from build123d import *

# Parameters (mm, degrees)
BOSS_EXTRUDE1_DEPTH = 10
BOSS_EXTRUDE2_DEPTH = 20
BOSS_EXTRUDE3_REACH = 38.449
FILLET1_R           = 1
CUT_EXTRUDE1_DEPTH  = 7


with BuildPart() as part:
    # Sketch1 → Boss-Extrude1 (new body)
    with BuildSketch(Plane(origin=(0, 0, 0), x_dir=(1, 0, 0), z_dir=(0, 1, 0))):
        Polygon((15, 0), (12.135254916, 8.816778784), (4.635254916, 14.265847744), (-4.635254916, 14.265847744), (-12.135254916, 8.816778784), (-15, 0), (-12.135254916, -8.816778784), (-4.635254916, -14.265847744), (4.635254916, -14.265847744), (12.135254916, -8.816778784), align=None)
    extrude(amount=BOSS_EXTRUDE1_DEPTH)

    # Sketch2 → Boss-Extrude2 (add)
    with BuildSketch(Plane(origin=(0, 10, 0), x_dir=(1, 0, 0), z_dir=(0, 1, 0))):
        Polygon((10, 0), (8.090169944, 5.877852523), (3.090169944, 9.510565163), (-3.090169944, 9.510565163), (-8.090169944, 5.877852523), (-10, 0), (-8.090169944, -5.877852523), (-3.090169944, -9.510565163), (3.090169944, -9.510565163), (8.090169944, -5.877852523), align=None)
    extrude(amount=BOSS_EXTRUDE2_DEPTH)

    # Boss-Extrude3: up to this face of the body (flat: up to its plane)
    boss_extrude3_end = Plane(part.part.faces().sort_by_distance((0, 0, 0))[0])
    # Sketch3 → Boss-Extrude3 (add, up to the picked face)
    with BuildSketch(Plane(origin=(0, 30, 0), x_dir=(1, 0, 0), z_dir=(0, 1, 0)), mode=Mode.PRIVATE) as boss_extrude3_sk1:
        Polygon((-16.180339887, 11.755705046), (-10, 0), (-8.090169944, 5.877852523), align=None)
    boss_extrude3_tool1 = split(extrude(boss_extrude3_sk1.sketch, amount=-BOSS_EXTRUDE3_REACH, mode=Mode.PRIVATE), bisect_by=boss_extrude3_end, keep=Keep.BOTH, mode=Mode.PRIVATE)
    # Sketch3 → Boss-Extrude3 (add, up to the picked face)
    with BuildSketch(Plane(origin=(0, 30, 0), x_dir=(1, 0, 0), z_dir=(0, 1, 0)), mode=Mode.PRIVATE) as boss_extrude3_sk2:
        Polygon((-3.090169944, 9.510565163), (-16.180339887, 11.755705046), (-8.090169944, 5.877852523), align=None)
    boss_extrude3_tool2 = split(extrude(boss_extrude3_sk2.sketch, amount=-BOSS_EXTRUDE3_REACH, mode=Mode.PRIVATE), bisect_by=boss_extrude3_end, keep=Keep.BOTH, mode=Mode.PRIVATE)
    add(boss_extrude3_tool1.solids().sort_by(Axis((-11.423503, 30, -5.877853), (0, -1, 0)))[0])
    add(boss_extrude3_tool2.solids().sort_by(Axis((-9.120227, 30, -9.048041), (0, -1, 0)))[0])

    # Fillet1
    fillet1_edges = [part.edges().sort_by_distance(p)[0] for p in [
        (8.385254916, 10, -11.541313264),
        (0, 10, -14.265847744),
        (-7.135254916, 10, -12.449491424),
        (-13.567627458, 10, 4.408389392),
        (-8.385254916, 10, 11.541313264),
        (0, 10, 14.265847744),
        (9.045084972, 30, 2.938926261),
        (9.045084972, 30, -2.938926261),
        (5.590169944, 30, -7.694208843),
        (0, 30, -9.510565163),
        (-9.045084972, 30, 2.938926261),
        (-5.590169944, 30, 7.694208843),
        (0, 30, 9.510565163),
        (5.590169944, 30, 7.694208843),
        (8.385254916, 10, 11.541313264),
        (13.567627458, 10, 4.408389392),
        (-14.045084972, 10, -2.938926261),
        (-16.180339887, 15, -11.755705046),
        (-9.635254916, 30, -10.633135104),
        (-13.090169944, 30, -5.877852523),
        (13.567627458, 10, -4.408389392),
    ]]
    fillet(fillet1_edges, radius=FILLET1_R)

    # Sketch4 → Cut-Extrude1 (cut)
    with BuildSketch(Plane(origin=(0, 0, 0), x_dir=(-1, 0, 0), z_dir=(0, -1, 0))):
        with BuildLine():
            ThreePointArc((3.45, 0), (3.281144981, 1.066108631), (2.791108631, 2.02785912))
            Line((2.791108631, 2.02785912), (-1.253976341, -0.911067141))
            Line((-1.253976341, -0.911067141), (0.557699479, -3.404624985))
            ThreePointArc((0.557699479, -3.404624985), (2.629312001, -2.233655837), (3.45, 0))
        make_face()
        with BuildLine():
            Line((-1.253976341, -0.911067141), (2.791108631, 2.02785912))
            ThreePointArc((2.791108631, 2.02785912), (-0.261594714, 3.440068052), (-3.065652161, 1.582490703))
            Line((-3.065652161, 1.582490703), (-1.253976341, -0.911067141))
        make_face()
    extrude(amount=-CUT_EXTRUDE1_DEPTH, mode=Mode.SUBTRACT)


solid = part.part
Work out the finished part from the listing and answer in its coordinate system (mm). A direction names the side the tool comes from. Give positions to 0.01 mm unless a question says otherwise; leave off trailing zeros. Loops run counter-clockwise (first coordinate to the right, second up) from the corner with the lowest first, then second, coordinate; pieces in that order, holes last. Notation, with made-up numbers: (69.25, 61.5) -> (88.25, 61.5) arc R32 cw to (88.25, 87.5) -> close; hole circle Ø7 at (83, 69.25). An arc over 180 degrees is marked (long way). Use a Markdown table: item, result. Add a question column.
1. Section B-B on x = 0 is taken. Determine the outline of the cut face in (y, z).
2. Determine the mould class of faces 4 (the flat face through (-5.625, 19.367, 7.669)), 5 (the flat face through (-14.03, 4.44, -2.98)), 6 (the flat face through (9.23, 10, 2.89)) for opening direction Z: released by +Z, released by -Z, zero draft, split by the parting line, or undercut.
3. For faces 1 (the flat face through (1.279, 3.451, 0.876)), 2 (the flat face through (5.555, 19.367, 7.72)), 3 (the cylindrical face through (-0.086, 29.715, -9.21)), determine the directions among +Z, -Z, +X, -X, +Y, -Y from which every point of the face is accessible in a straight line to the end or side of a thin tool.
4. Flat-ended cylindrical pins translate along their axes: pin 1 Ø1.9 at (x, y) = (-0.5, 18.5) entering from -Z; pin 2 Ø12 at (x, y) = (11.5, 11) entering from +Z; pin 3 Ø5 at (x, y) = (-1, 19.5) entering from +Z. Find the tip coordinate at first contact, or state that the pin passes through.
5. Find the intervals of material crossed by probe 1 along Y at (x, z) = (-3, 11.25); probe 2 along Z at (x, y) = (-3, 26); probe 3 along X at (y, z) = (20.5, -2.75), in increasing order.
6. Section A-A on y = 11.5 is taken. Determine the outline of the cut face in (x, z), and give its area (3 significant figures).
Results below:
| question | item | result |
|---|---|---|
| 1 | outline | (0, -14.27) -> (9, -14.27) arc R1 ccw to (10, -13.27) -> (10, -9.51) -> (29, -9.51) arc R1 ccw to (30, -8.51) -> (30, 8.51) arc R1 ccw to (29, 9.51) -> (10, 9.51) -> (10, 13.27) arc R1 ccw to (9, 14.27) -> (0, 14.27) -> (0, 2.64) -> (7, 2.64) -> (7, -3.45) -> (0, -3.45) -> close |
| 2 | face 4 | released by +Z |
| 2 | face 5 | undercut |
| 2 | face 6 | zero draft |
| 3 | face 1 | -Y |
| 3 | face 2 | +Z, +X, +Y |
| 3 | face 3 | -Z, +X, +Y |
| 4 | pin 1 | stops at z = -9.51 |
| 4 | pin 2 | stops at z = 13.41 |
| 4 | pin 3 | stops at z = 9.51 |
| 5 | probe 1 | y = 0 to 10 |
| 5 | probe 2 | z = -9.51 to 9.51 |
| 5 | probe 3 | x = -11.45 to 9.11 |
| 6 | outline | (-15.24, -9.96) arc R1 ccw to (-14.18, -11.41) -> (-3.09, -9.51) -> (3.09, -9.51) -> (8.09, -5.88) -> (10, 0) -> (8.09, 5.88) -> (3.09, 9.51) -> (-3.09, 9.51) -> (-8.09, 5.88) -> (-10, 0) -> close |
| 6 | area | 352 mm^2 |
